Input: part model. Units: mm. Frame: model coordinates. Face numbers are marked on the shaded views. A direction names the side the tool comes from. Give positions to 0.01 mm unless a question says otherwise; leave off trailing zeros. Order: outer loops, then holes, each group sorted by start corner. A loop starts at its lowest first (then second) coordinate and runs counter-clockwise, first axis right, second up. Notation, with made-up numbers: (4, 37) - (56, 37) arc R21 ccw to (56, 75) - close; hole circle Ø10 at (86.25, 11.5). An arc over 180 degrees is marked (long way). Use a Markdown table: item, result.
from build123d import *

# Parameters (mm, degrees)
ESQUISSE1_W          = 30
ESQUISSE1_H          = 40
BASE_EXTRUSION_DEPTH = 8
ESQUISSE2_W          = 10
ESQUISSE2_H          = 34
BOSS_EXTRU_1_DEPTH   = 20
ESQUISSE3_R          = 11.25
BOSS_EXTRU_2_DEPTH   = 14


with BuildPart() as part:
    # Esquisse1 → Base-Extrusion (new body)
    with BuildSketch(Plane.XY):
        Rectangle(ESQUISSE1_W, ESQUISSE1_H)
    extrude(amount=BASE_EXTRUSION_DEPTH)

    # Esquisse2 → Boss.-Extru.1 (add)
    with BuildSketch(Plane(origin=(0, 0, 0), x_dir=(-1, 0, 0), z_dir=(0, 0, -1))):
        Rectangle(ESQUISSE2_W, ESQUISSE2_H)
    extrude(amount=BOSS_EXTRU_1_DEPTH)

    # Esquisse3 → Boss.-Extru.2 (add)
    with BuildSketch(Plane.XY.offset(8)):
        Circle(ESQUISSE3_R)
    extrude(amount=BOSS_EXTRU_2_DEPTH)


solid = part.part
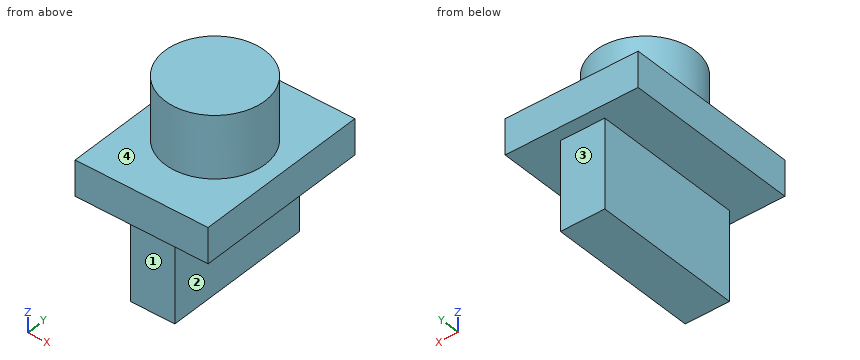
1. Section query C-C (z = 16). Return loops of the section in (x, y).
Response:
| item | result |
|---|---|
| outline | circle Ø22.5 at (0, 0) |
2. Section query A-A (y = 0). Return loops of the section in (x, z), then the cut area to 3 significant figures.
Response:
| item | result |
|---|---|
| outline | (-15, 0) - (-5, 0) - (-5, -20) - (5, -20) - (5, 0) - (15, 0) - (15, 8) - (11.25, 8) - (11.25, 22) - (-11.25, 22) - (-11.25, 8) - (-15, 8) - close |
| area | 755 mm^2 |
3. Set-up query: the marked faces 1, 2, 3 and 4. Return all of +Z, -Z, +X, -X, +Y, -Y with unobstructed straight access to the full face (end or side cutting, diameter ignored); none if empty.
Response:
| item | result |
|---|---|
| face 1 | -Z, +X, -X, -Y |
| face 2 | -Z, +X, +Y, -Y |
| face 3 | -Z, +X, -X, +Y |
| face 4 | +Z |
4. Material intervals for line 1 along Y through (x, z) = (2.5, -9); line 2 along X through (y, z) = (-4, -11); line 3 along Z through (x, y) = (5.75, 7.5), sorted ascending.
Response:
| item | result |
|---|---|
| line 1 | y = -17 to 17 |
| line 2 | x = -5 to 5 |
| line 3 | z = 0 to 22 |
5. Pin query (flat end, axial travel): pin 1 (1.5 mm diameter, centred on x = -0.5, z = 15, fed in from +Y); pin 2 (6 mm diameter, centred on y = 2.5, z = -8.5, fed in from -X); pin 3 (5 mm diameter, centred on x = -1.5, z = -7, fed in from -Y). Return the tip coordinate at first contact, or that it passes through.
Response:
| item | result |
|---|---|
| pin 1 | stops at y = 11.25 |
| pin 2 | stops at x = -5 |
| pin 3 | stops at y = -17 |
6. Section query D-D (y = -15). Return loops of the section in (x, z), then the cut area to 3 significant figures.
Response:
| item | result |
|---|---|
| outline | (-15, 0) - (-5, 0) - (-5, -20) - (5, -20) - (5, 0) - (15, 0) - (15, 8) - (-15, 8) - close |
| area | 440 mm^2 |
7. Section query B-B (x = 0). Return loops of the section in (y, z), then the cut area to 4 significant figures.
Response:
| item | result |
|---|---|
| outline | (-20, 0) - (-17, 0) - (-17, -20) - (17, -20) - (17, 0) - (20, 0) - (20, 8) - (11.25, 8) - (11.25, 22) - (-11.25, 22) - (-11.25, 8) - (-20, 8) - close |
| area | 1,315 mm^2 |
